Geometry check sheet. Reference: drawing and pictorial views, mm from the part's lowest x, y, z. Round coordinates to 2 decimals unless told otherwise and drop trailing zeros. Write each loop counter-clockwise with the first axis right and the second up, starting at its lowest first coordinate (ties: lowest second). Pieces come first, ordered by that corner, then holes. Notation, with made-up numbers: M 43.25,17 L 62.25,17 A28 ccw 62.25,56 Z; hole C 14.25,4.25 d4. An arc over 180 degrees is marked long. Use a Markdown table: item, result. Add a question column.
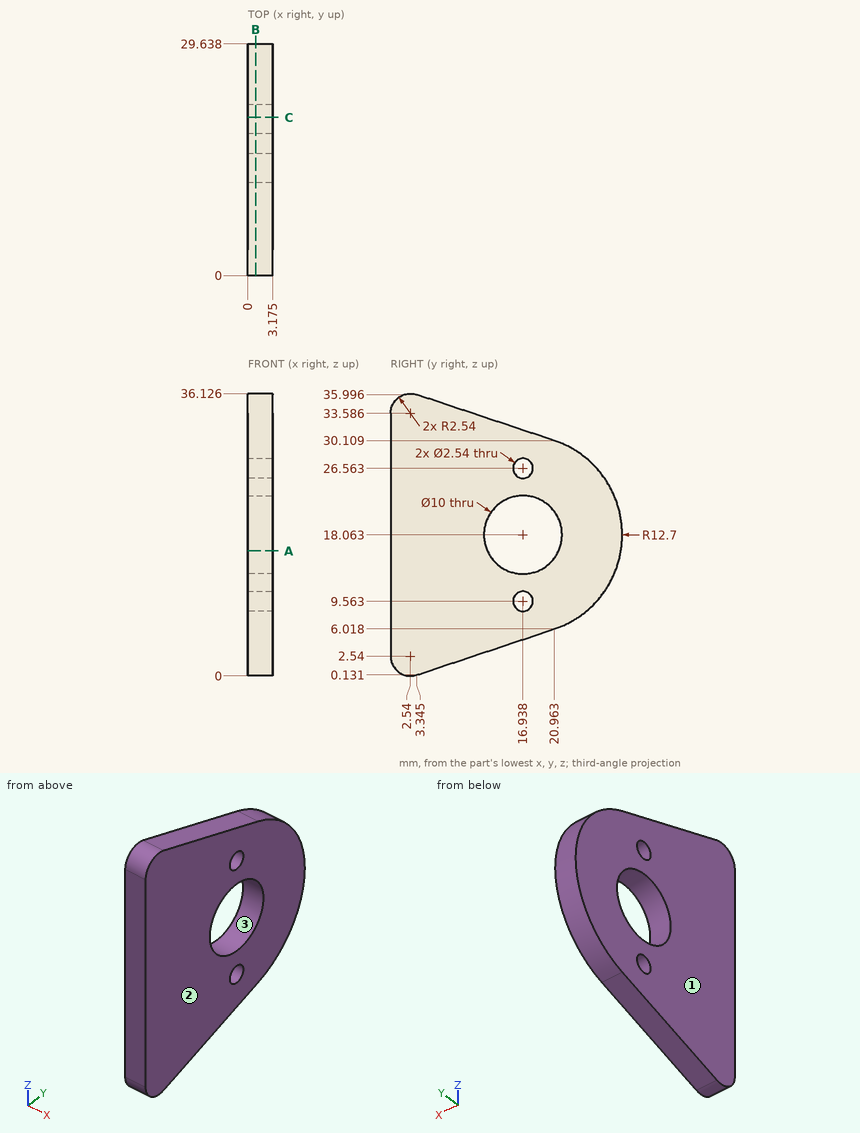
1. Cross-section at B-B on x = 1. Enter the section's corners in (y, z) (1 decimal).
2. Cross-section at C-C on y = 20.25. Enter the section's corners in (x, z) (1 decimal).
3. Cross-section at A-A on z = 16. Enter the section's corners in (x, y) (1 decimal).
4. Release check for a two-part mould opening along X. For the marked faces 1, 2 and 3 record: +X half, -X half, draft (parallel to the pull), parting line (faces both ways), or undercut.
5. Scan lines: line 1 along Y through (x, z) = (1.7, 15.5) (1 decimal); line 2 along Z through (x, y) = (2.25, 15) (1 decimal); line 3 along Y through (x, z) = (0.7, 15) (1 decimal). Record each from-to range of solid material in increasing order. Write a range as from..to.
6. Depth check by flat-ended pin: pin 1 Ø1 at (x, y) = (0.5, 26.5) entering from +Z; pin 2 Ø2 at (y, z) = (16.94, 9.56) entering from +X; pin 3 Ø13 at (y, z) = (16.94, 18.06) entering from +X (1 decimal). Enter the tip coordinate at first touch or a pass-through.
Answer:
| question | item | result |
|---|---|---|
| 1 | outline | M 0,2.5 A2.5 ccw 3.3,0.1 L 21,6 A12.7 ccw 21,30.1 L 3.3,36 A2.5 ccw 0,33.6 Z; hole C 16.9,18.1 d10; hole C 16.9,9.6 d2.5; hole C 16.9,26.6 d2.5 |
| 2 | outline | M 0,5.8 L 3.2,5.8 L 3.2,14.3 L 0,14.3 Z; M 0,21.8 L 3.2,21.8 L 3.2,30.3 L 0,30.3 Z |
| 3 | outline | M 0,0 L 3.2,0 L 3.2,12.4 L 0,12.4 Z; M 0,21.5 L 3.2,21.5 L 3.2,29.5 L 0,29.5 Z |
| 4 | face 1 | -X half |
| 4 | face 2 | +X half |
| 4 | face 3 | draft |
| 5 | line 1 | y = 0..12.6, 21.2..29.4 |
| 5 | line 2 | z = 4..13.5, 22.7..32.1 |
| 5 | line 3 | y = 0..13, 20.9..29.3 |
| 6 | pin 1 | stops at z = 26.96 |
| 6 | pin 2 | passes through |
| 6 | pin 3 | stops at x = 3.2 |
